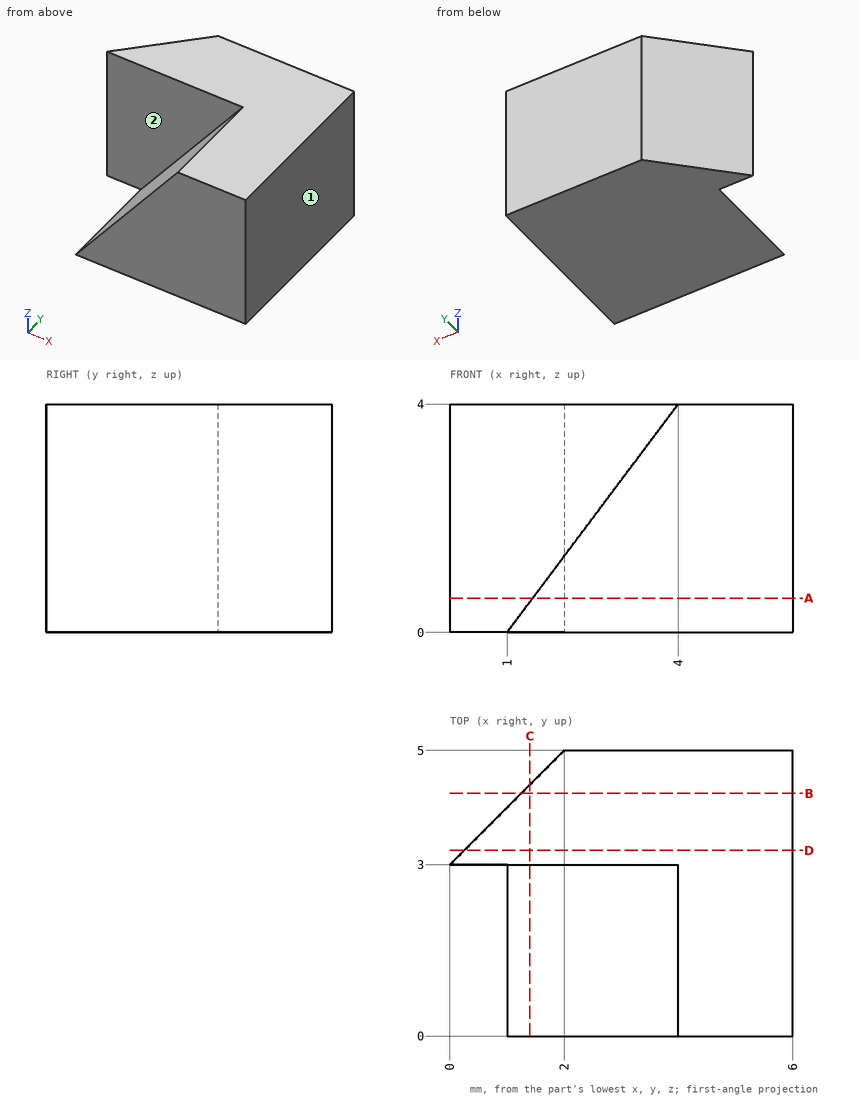
Could you check a few things on this drawing? It's one solid part, dimensions in mm from its lowest x, y, z. A direction names the side the tool comes from. Give positions to 0.01 mm unless a question says otherwise; leave off trailing zeros. Write each loop counter-clockwise with the first axis right and the second up, starting at its lowest first coordinate (ties: lowest second). Pieces come first, ordered by that corner, then holes. Notation, with made-up numbers: M -30,-19.5 L 22,-19.5 A11 ccw 22,-15.5 Z; hole C 22,32.5 d5. An arc over 180 degrees is marked long. Put each result on its own line as item: value. Start each with the question number.
Item 1: If we section it at C-C, the plane x = 1.4: Write out the boundary of the cut face in (y, z), then the cut area to 3 significant figures.
Item 2: If we section it at D-D, the plane y = 3.25: Write out the boundary of the cut face in (x, z), then the cut area to 3 significant figures.
Item 3: Will this pin go through, and if not, where does the flat tip stop? pin 1 (1.5 mm diameter, centred on y = 0.5, z = 2.5, fed in from -X).
Item 4: If we section it at B-B, the plane y = 4.25: Write out the boundary of the cut face in (x, z).
Item 5: If we section it at A-A, the plane z = 0.6: Write out the boundary of the cut face in (x, y), then the cut area to 4 significant figures.
Item 6: I need wall thicknesses on L1, parallel to Y at x = 2.3, z = 3.1; L2, parallel to X at y = 4, z = 1.3; L3, parallel to X at y = 2.6, z = 0.85. Which ranges of each line are inside material? Lowest first, please. Write a range as from..to.
Item 7: On a 3-axis mill with a long thin cutter (end or side, diameter ignored), from which of +Z, -Z, +X, -X, +Y, -Y can I reach the whole of each face in a straight line? I mean the marked faces 1 and 2. Say none if no direction works.
Values:
1. outline: M 0,0 L 4.4,0 L 4.4,4 L 3,4 L 3,0.53 L 0,0.53 Z
1. area: 7.20 mm²
2. outline: M 0.25,0 L 6,0 L 6,4 L 0.25,4 Z
2. area: 23.0 mm²
3. pin 1: x = 2.31
4. outline: M 1.25,0 L 6,0 L 6,4 L 1.25,4 Z
5. outline: M 0,3 L 1.45,3 L 1.45,0 L 6,0 L 6,5 L 2,5 Z
5. area: 23.65 mm²
6. L1: 3..5
6. L2: 1..6
6. L3: 1.64..6
7. face 1: +Z, -Z, +X, +Y, -Y
7. face 2: +Z, -X, -Y
